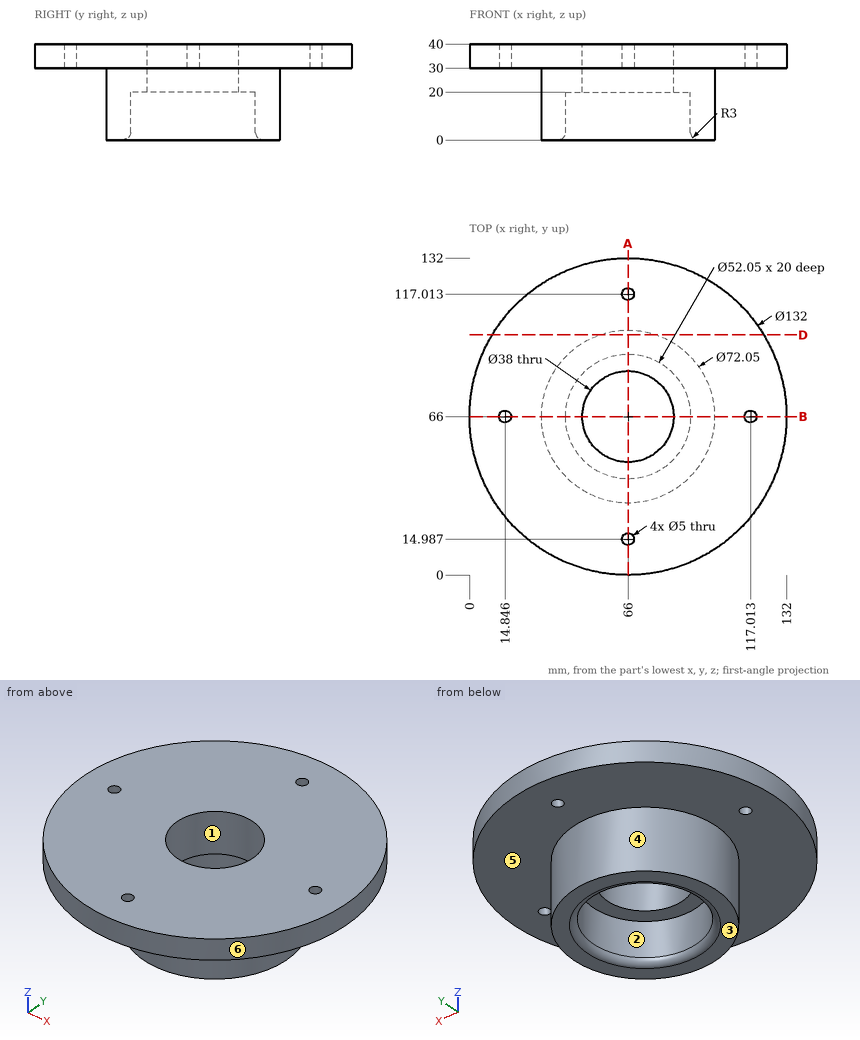
Source: three-view drawing plus pictorial views. Frame: mm from the lowest corner of the part. A direction names the side the tool comes from. Round coordinates to 2 decimals unless told otherwise and drop trailing zeros. Write each loop counter-clockwise with the first axis right and the second up, starting at its lowest first coordinate (ties: lowest second). Pieces come first, ordered by that corner, then holes. Notation, with made-up numbers: M 76.5,14 L 115.5,14 A29 ccw 115.5,44 Z; hole C -31,30 d1. An arc over 180 degrees is marked long. Use CSV: the item, a comma, the result in double quotes. Start each with the question number.
Q1. Cut plane A-A on x = 66. Output: boundary loops of the cut face in (y, z) (1 decimal), plus the area to 3 significant figures.
Q2. Pull-direction query (X, two-part tool) for the marked faces 1, 2, 3 and 4; classes: +X half, -X half, draft (parallel to the pull), parting line (faces both ways), or undercut.
Q3. First-contact query: P1, Ø6, axis at x = 99.5, z = 15, coming from the +Y side; P2, Ø8, axis at y = 88.5, z = 18, coming from the +X side; P3, Ø1, axis at x = 51.5, z = 15, coming from the +Y side. Flat tips, straight axial feed; report the tip coordinate or a pass-through.
Q4. Access query for the marked faces 5 and 6. Directions: +Z, -Z, +X, -X, +Y, -Y. A direction counts if a zero-diameter tool reaches every point of the face in a straight line with its end or side. Return the directions, or none.
Q5. Cut plane B-B on y = 66. Output: boundary loops of the cut face in (x, z) (1 decimal), plus the area to 3 significant figures.
Q6. Cut plane D-D on y = 100. Output: boundary loops of the cut face in (x, z).
Q7. Line query: line 1 (Y direction, x = 66, z = 35); line 2 (X direction, y = 65.5, z = 36) (1 decimal); line 3 (X direction, y = 74, z = 7) (1 decimal). Output: solid intervals per line, ascending. Write a range as from..to.
Results found:
1,outline,"M 0,30 L 12.5,30 L 12.5,40 L 0,40 Z; M 17.5,30 L 30,30 L 30,0 L 37,0 A3 ccw 40,3 L 40,20 L 47,20 L 47,40 L 17.5,40 Z; M 85,20 L 92,20 L 92,3 A3 ccw 95,0 L 102,0 L 102,30 L 114.5,30 L 114.5,40 L 85,40 Z; M 119.5,30 L 132,30 L 132,40 L 119.5,40 Z"
1,area,"1,580 mm^2"
2,face 1,"undercut"
2,face 2,"undercut"
2,face 3,"draft"
2,face 4,"parting line"
3,P1,"y = 85.17"
3,P2,"x = 96.91"
3,P3,"y = 99.19"
4,face 5,"-Z"
4,face 6,"+Z, -Z"
5,outline,"M 0,30 L 12.3,30 L 12.3,40 L 0,40 Z; M 17.3,30 L 30,30 L 30,0 L 37,0 A3 ccw 40,3 L 40,20 L 47,20 L 47,40 L 17.3,40 Z; M 85,20 L 92,20 L 92,3 A3 ccw 95,0 L 102,0 L 102,30 L 114.5,30 L 114.5,40 L 85,40 Z; M 119.5,30 L 132,30 L 132,40 L 119.5,40 Z"
5,area,"1,580 mm^2"
6,outline,"M 9.43,30 L 54.09,30 L 54.09,0 L 77.91,0 L 77.91,30 L 122.57,30 L 122.57,40 L 9.43,40 Z"
7,line 1,"0..12.49, 17.49..47, 85..114.51, 119.51..132"
7,line 2,"0..12.4, 17.3..47, 85..114.6, 119.5..132"
7,line 3,"30.9..41.2, 90.8..101.1"
